Answer from the drawing. Dimensions are ordinates in mm from the lowest x, y and z of the part. A direction names the side the tool comes from. Give positions to 0.01 mm unless a question says otherwise; leave off trailing zeros. Order: outer loops, then holes, each group sorted by start corner. A loop starts at its lowest first (then second) coordinate and runs counter-clockwise, first axis right, second up. Notation, with made-up numbers: (78, 25) - (137, 25) arc R22 ccw to (137, 37) - close; hole circle Ø10 at (48.25, 79.5). An arc over 180 degrees is marked (long way). One line per item, written item: value. Start each with the question number.
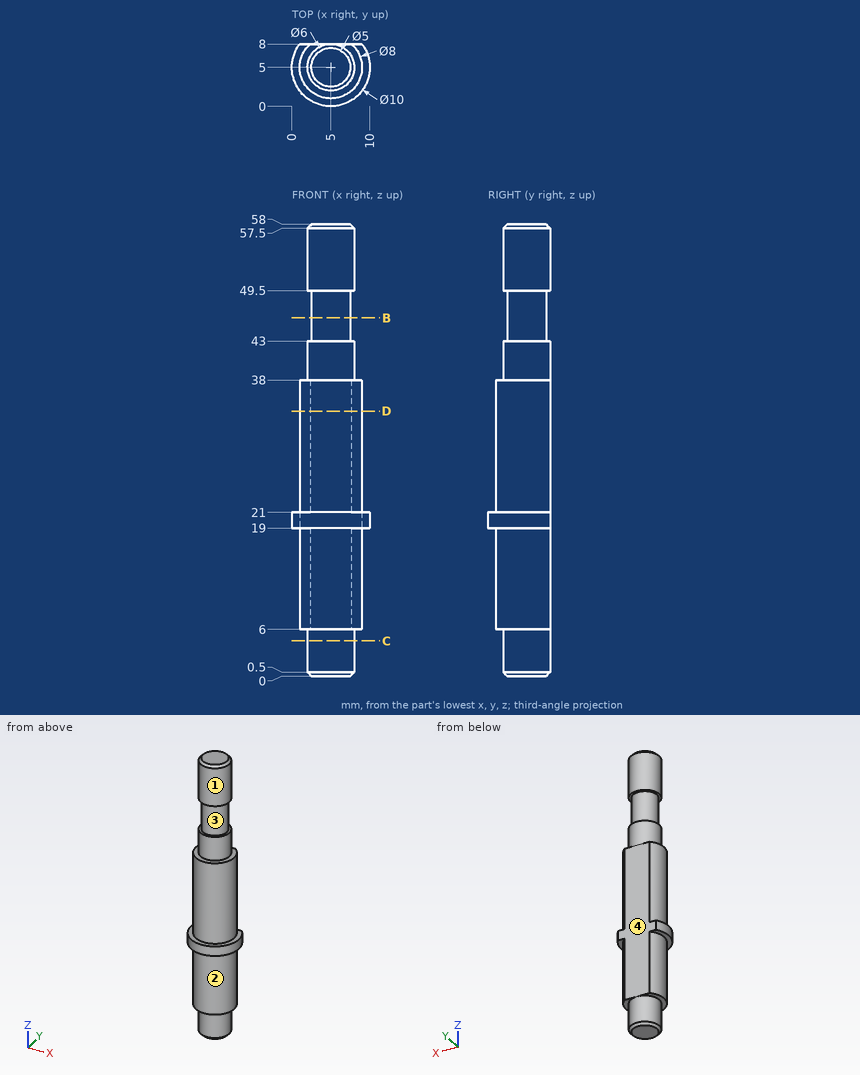
1) Section D-D on z = 34 is taken. Write down the section's boundary in (x, y), plus the area to 3 significant figures.
2) Section B-B on z = 46 is taken. Write down the section's boundary in (x, y).
3) Section C-C on z = 4.5 is taken. Write down the section's boundary in (x, y).
4) Each of these flat-tipped pins is pushed along its axis until it touches: pin 1 (1.8 mm diameter, centred on x = 4.5, y = 6, fed in from -Z); pin 2 (1 mm diameter, centred on x = 7.5, y = 7, fed in from -Z); pin 3 (4 mm diameter, centred on y = 5.5, z = 42.5, fed in from +X); pin 4 (1.5 mm diameter, centred on y = 6.5, z = 37, fed in from -X). Where does it stop, or does it pass through?
5) Find the intervals of material crossed by probe 1 along Z at (x, y) = (7, 1.75); probe 2 along Z at (x, y) = (6.75, 1); probe 3 along Z at (x, y) = (6.75, 2.75), in increasing order. Write a range as from..to.
6) For the marked faces 1 and 2, determine the directions among +Z, -Z, +X, -X, +Y, -Y from which every point of the face is accessible in a straight line to the end or side of a thin tool.
7) The mould has two halves that part along Z. Classify the marked faces 3 and 4: +Z half, -Z half, draft (parallel to the pull), parting line (faces both ways), or undercut.
Solved:
1. outline: (2.35, 8) arc R4 ccw (long way) to (7.65, 8) - close
1. area: 46.6 mm2
2. outline: circle Ø5 at (5, 5)
3. outline: circle Ø6 at (5, 5)
4. pin 1: stops at z = 0
4. pin 2: stops at z = 0.2
4. pin 3: stops at x = 8
4. pin 4: stops at x = 1.07
5. probe 1: z = 6..38
5. probe 2: z = 19..21
5. probe 3: z = 0.35..43, 49.5..57.65
6. face 1: +Z
6. face 2: -Z
7. face 3: undercut
7. face 4: draft
